```python
from build123d import *

# Parameters (mm, degrees)
SKETCH2_R           = 5.264069535
BOSS_EXTRUDE1_DEPTH = 0.7
SKETCH3_W           = 0.5
SKETCH3_H           = 2
BOSS_EXTRUDE2_DEPTH = 3.9


with BuildPart() as part:
    # Sketch1 → Revolve1 (revolve)
    with BuildSketch(Plane.XY):
        Polygon((0, -14.9), (6, -14.9), (6, 0), (7, 0), (5.043279744, 1.45), (4.6, 1.45), (4.6, 2.9), (0, 2.9), align=None)
    revolve(axis=Axis((0, 2.9, 0), (0, -1, 0)))

    # Sketch2 → Boss-Extrude1 (add)
    with BuildSketch(Plane.XZ.offset(14.9)):
        Circle(SKETCH2_R)
    extrude(amount=BOSS_EXTRUDE1_DEPTH)

    # Sketch3 → Boss-Extrude2 (add)
    with BuildSketch(Plane.XZ.offset(15.6)):
        with Locations((-3.65, 0)):
            Rectangle(SKETCH3_W, SKETCH3_H)
        with Locations((3.65, 0)):
            Rectangle(SKETCH3_W, SKETCH3_H)
    extrude(amount=BOSS_EXTRUDE2_DEPTH)


solid = part.part
```
Input: part model. Units: mm. Frame: model coordinates. A direction names the side the tool comes from. Give positions to 0.01 mm unless a question says otherwise; leave off trailing zeros. Order: outer loops, then holes, each group sorted by start corner. A loop starts at its lowest first (then second) coordinate and runs counter-clockwise, first axis right, second up. Notation, with made-up numbers: M 71,70 L 115,70 A30 ccw 115,104 Z; hole C -28.5,25 d11. An arc over 180 degrees is marked long. One line per question, with ' | ' between items. Start each with the question number.
1. Material intervals for probe 1 along Y at (x, z) = (-0.25, -0.5); probe 2 along Z at (x, y) = (1, -1.5); probe 3 along Z at (x, y) = (5.25, -12.25), sorted ascending. Write a range as [from, to].
2. First-contact query: pin 1 Ø2 at (y, z) = (-8.5, -5.5) entering from -X; pin 2 Ø2 at (y, z) = (-17.5, 0) entering from -X; pin 3 Ø1.5 at (x, z) = (-5, -3.5) entering from -Y. Flat tips, straight axial feed; report the tip coordinate or a pass-through.
3. Section query B-B (x = 0). Return the cut outline in (y, z), and give its area (3 significant figures).
4. Section query A-A (y = -16.5). Return the cut outline in (x, z), and give its area (3 significant figures).
5. Section query D-D (y = -11.25). Return the cut outline in (x, z).
6. Section query C-C (z = 0). Return the cut outline in (x, y).
7. Pull-direction query (Z, two-part tool) for faces 6 (the face through (-6, 0, 2)), 7 (the face through (5.02, -15.25, 1.58)); classes: released by +Z, released by -Z, zero draft, split by the parting line, or undercut.
8. Access query for faces 1 (the face through (3.4, -18, 0)), 2 (the face through (-3.9, -18, 0)), 3 (the face through (-6, -7, 0)), 4 (the face through (-3.65, 2.19, -2.8)), 5 (the face through (3.9, -18, 0)). Directions: +Z, -Z, +X, -X, +Y, -Y. A direction counts if a zero-diameter tool reaches every point of the face in a straight line with its end or side. Return the directions, or none.
Here are the results:
1) probe 1: [-15.6, 2.9] | probe 2: [-5.92, 5.92] | probe 3: [-2.9, 2.9]
2) pin 1: x = -3.97 | pin 2: x = -3.9 | pin 3: y = -14.9
3) outline: M -15.6,-5.26 L -14.9,-5.26 L -14.9,-6 L 0,-6 L 0,-7 L 1.45,-5.04 L 1.45,-4.6 L 2.9,-4.6 L 2.9,4.6 L 1.45,4.6 L 1.45,5.04 L 0,7 L 0,6 L -14.9,6 L -14.9,5.26 L -15.6,5.26 Z | area: 217 mm²
4) outline: M -3.9,-1 L -3.4,-1 L -3.4,1 L -3.9,1 Z; M 3.4,-1 L 3.9,-1 L 3.9,1 L 3.4,1 Z | area: 2.00 mm²
5) outline: C 0,0 d12
6) outline: M -7,0 L -6,0 L -6,-14.9 L -5.26,-14.9 L -5.26,-15.6 L -3.9,-15.6 L -3.9,-19.5 L -3.4,-19.5 L -3.4,-15.6 L 3.4,-15.6 L 3.4,-19.5 L 3.9,-19.5 L 3.9,-15.6 L 5.26,-15.6 L 5.26,-14.9 L 6,-14.9 L 6,0 L 7,0 L 5.04,1.45 L 4.6,1.45 L 4.6,2.9 L -4.6,2.9 L -4.6,1.45 L -5.04,1.45 Z
7) face 6: zero draft | face 7: split by the parting line
8) face 1: +Z, -Z, -Y | face 2: +Z, -Z, -X, -Y | face 3: -Y | face 4: +Y | face 5: +Z, -Z, +X, -Y
